Could you check a few things on this model? Use its own coordinates, in mm. A direction names the side the tool comes from. Give positions to 0.01 mm unless a question says otherwise; leave off trailing zeros. Write each loop counter-clockwise with the first axis right and the second up, starting at its lowest first coordinate (ties: lowest second). Pieces come first, ordered by that corner, then holes. Notation, with made-up numbers: (10.25, -35.5) - (20.25, -35.5) arc R10 cw to (20.25, -23.5) - close; hole circle Ø4 at (10.25, 76). An arc over 180 degrees is marked (long way). Write item = value, one per line.
Solid Edge part; units mm, degrees
sketch "Sketch1" plane through (0, 0, 8) normal (0, 0, 1) x (1, 0, 0)
  circle A0 centre (0, 0) radius 21
  circle A1 centre (0, 0) radius 12
  circle A2 centre (11.3137, 11.3137) radius 1.7
  circle A3 centre (-11.3137, 11.3137) radius 1.7
  circle A4 centre (-11.3137, -11.3137) radius 1.7
  circle A5 centre (11.3137, -11.3137) radius 1.7
extrude "ExtrudedProtrusion_1" add sketch "Sketch1" along normal blind 4
sketch "Sketch2" plane through (0, 0, 8) normal (0, 0, 1) x (1, 0, 0)
  line L0 (12, -12) -> (73, -12)
  line L1 (73, -12) -> (73, 12)
  line L2 (73, 12) -> (12, 12)
  line L3 (12, 12) -> (12, -12)
extrude "ExtrudedProtrusion_2" add sketch "Sketch2" along normal blind 4
sketch "Sketch3" plane through (0, 0, 8) normal (0, 0, 1) x (1, 0, 0)
  line L0 (57, -49) -> (113, -49)
  line L1 (113, -49) -> (113, 24)
  line L2 (113, 24) -> (57, 24)
  line L3 (57, 24) -> (57, -49)
  circle A0 centre (62, -43) radius 1.7
  circle A1 centre (108, -43) radius 1.7
  circle A2 centre (62, 18) radius 1.7
  circle A3 centre (108, 18) radius 1.7
extrude "ExtrudedProtrusion_3" add sketch "Sketch3" along normal blind 4
sketch "Sketch4" plane through (0, 0, 8) normal (0, 0, 1) x (1, 0, 0)
  circle A0 centre (11.3137, 11.3137) radius 1.7
  circle A1 centre (-11.3137, 11.3137) radius 1.7
  circle A2 centre (-11.3137, -11.3137) radius 1.7
  circle A3 centre (11.3137, -11.3137) radius 1.7
  circle A4 centre (62, -43) radius 1.7
  circle A5 centre (108, -43) radius 1.7
  circle A6 centre (62, 18) radius 1.7
  circle A7 centre (108, 18) radius 1.7
extrude "ExtrudedCutout_1" cut sketch "Sketch4" along normal blind 4
1. Thinking about a two-plate mould opening in X: for faces 1 (the face through (85, 24, 10)), 2 (the face through (-11.99, -0.53, 9.97)), 3 (the face through (60.3, 17.93, 9.97)), 4 (the face through (113, -13, 10)), which applies, pulls with the +X half, pulls with the -X half, needs draft (parallel to the pull), parting line crosses it, or undercut?
Filled sheet:
face_1 = needs draft
face_2 = undercut
face_3 = undercut
face_4 = pulls with the +X half
2. If we section it at A-A, the plane y = 0: Please give me the cut outline in (x, z), and give its area (3 significant figures).
Filled sheet:
outline = (-21, 8) - (-12, 8) - (-12, 12) - (-21, 12) - close; (12, 8) - (113, 8) - (113, 12) - (12, 12) - close
area = 440 mm2
3. For pin 1 (2 mm diameter, centred on x = 11.31, y = -11.31, fed in from +Z); pin 2 (1.2 mm diameter, centred on y = 17.5, z = 10.5, fed in from -X); pin 3 (1 mm diameter, centred on x = 4.5, z = 9.5, fed in from -Y); pin 4 (2 mm diameter, centred on x = 6.5, z = 10.5, fed in from -Y), each with a flat end and sliding along its axis, tell me the tip position at first contact or that it passes through.
Filled sheet:
pin_1 = through
pin_2 = -12.47
pin_3 = -20.62
pin_4 = -20.27
4. If we section it at B-B, the plane x = 0: Please give me the cut outline in (y, z).
Filled sheet:
outline = (-21, 8) - (-12, 8) - (-12, 12) - (-21, 12) - close; (12, 8) - (21, 8) - (21, 12) - (12, 12) - close
5. Which directions (+Z, -Z, +X, -X, +Y, -Y) give clear straight access to the entire face, cutting with the end or side of a thin tool? Please do faces 5 (the face through (37, 12, 10)), 6 (the face through (37, -12, 10)), 7 (the face through (85, -49, 10)).
Filled sheet:
face_5 = +Z, -Z, +Y
face_6 = +Z, -Z, -Y
face_7 = +Z, -Z, +X, -X, -Y
6. If we section it at D-D, the plane y = -43: Please give me the cut outline in (x, z), and give its area (3 significant figures).
Filled sheet:
outline = (57, 8) - (60.3, 8) - (60.3, 12) - (57, 12) - close; (63.7, 8) - (106.3, 8) - (106.3, 12) - (63.7, 12) - close; (109.7, 8) - (113, 8) - (113, 12) - (109.7, 12) - close
area = 197 mm2
7. I need wall thicknesses on line 1 (Y direction, x = 62, z = 9.6); line 2 (X direction, y = -44.5, z = 8.95); line 3 (Y direction, x = 61.5, z = 10.9). Which ranges of each line are inside material? Lowest first, please.
Filled sheet:
line_1 = -49 to -44.7, -41.3 to 16.3, 19.7 to 24
line_2 = 57 to 61.2, 62.8 to 107.2, 108.8 to 113
line_3 = -49 to -44.62, -41.38 to 16.38, 19.62 to 24
8. If we section it at C-C, the plane x = 62: Please give me the cut outline in (y, z).
Filled sheet:
outline = (-49, 8) - (-44.7, 8) - (-44.7, 12) - (-49, 12) - close; (-41.3, 8) - (16.3, 8) - (16.3, 12) - (-41.3, 12) - close; (19.7, 8) - (24, 8) - (24, 12) - (19.7, 12) - close
